Geometry check sheet. Reference: the model listing, model coordinates, mm. A direction names the side the tool comes from. Round coordinates to 2 decimals unless told otherwise and drop trailing zeros. Loops run counter-clockwise (first coordinate to the right, second up) from the corner with the lowest first, then second, coordinate; pieces in that order, holes last. Notation, with made-up numbers: (-7.75, 69) - (-3.75, 69) arc R23 cw to (-3.75, 84) - close; hole circle Ø10 at (85.5, 69.5). An arc over 180 degrees is marked (long way). Answer in a Markdown table with one row per item. Add a question column.
```python
from build123d import *

# Parameters (mm, degrees)
SKETCH1_W           = 151
SKETCH1_H           = 100
BOSS_EXTRUDE1_DEPTH = 105
SKETCH2_W           = 151
SKETCH2_H           = 100
SKETCH2_W_2         = 147
SKETCH2_H_2         = 96
CUT_EXTRUDE1_DEPTH  = 5
SKETCH3_W           = 20
SKETCH3_H           = 15
CUT_EXTRUDE2_DEPTH  = 2
SKETCH4_R           = 4
BOSS_EXTRUDE2_DEPTH = 5


with BuildPart() as part:
    # Sketch1 → Boss-Extrude1 (new body)
    with BuildSketch(Plane(origin=(0, 0, 0), x_dir=(1, 0, 0), z_dir=(0, 1, 0))):
        Rectangle(SKETCH1_W, SKETCH1_H)
    extrude(amount=BOSS_EXTRUDE1_DEPTH)

    # Sketch2 → Cut-Extrude1 (cut)
    with BuildSketch(Plane(origin=(0, 105, 0), x_dir=(1, 0, 0), z_dir=(0, 1, 0))):
        Rectangle(SKETCH2_W, SKETCH2_H)
        Rectangle(SKETCH2_W_2, SKETCH2_H_2, mode=Mode.SUBTRACT)
    extrude(amount=-CUT_EXTRUDE1_DEPTH, mode=Mode.SUBTRACT)

    # Sketch3 → Cut-Extrude2 (cut)
    with BuildSketch(Plane(origin=(0, 105, 0), x_dir=(1, 0, 0), z_dir=(0, 1, 0))):
        with Locations((63.5, 37.5)):
            Rectangle(SKETCH3_W, SKETCH3_H)
        with Locations((63.5, -37.5)):
            Rectangle(SKETCH3_W, SKETCH3_H)
    extrude(amount=-CUT_EXTRUDE2_DEPTH, mode=Mode.SUBTRACT)

    # Sketch4 → Boss-Extrude2 (add)
    with BuildSketch(Plane(origin=(0, 103, 0), x_dir=(1, 0, 0), z_dir=(0, 1, 0))):
        with Locations(Location((63.5, -37.5, 0), (0, 0, 270))):
            Circle(SKETCH4_R)
        with Locations(Location((63.5, 37.5, 0), (0, 0, 90))):
            Circle(SKETCH4_R)
    extrude(amount=BOSS_EXTRUDE2_DEPTH)


solid = part.part
```
Q1. Scan lines: line 1 (Y direction, x = 6, z = 23); line 2 (Y direction, x = 55.5, z = -32). Record each from-to range of solid material in increasing order. Write a range as from..to.
Q2. Cross-section at B-B, the plane z = -1. Enter the section's corners in (x, y).
Q3. Cross-section at A-A, the plane x = -21. Enter the section's corners in (y, z).
Q4. Depth check by flat-ended pin: P1, Ø5.5, axis at y = 103.5, z = -2, coming from the -X side; P2, Ø1.6, axis at y = 103.5, z = -41, coming from the +X side; P3, Ø0.6, axis at x = 61, y = 104, coming from the +Z side. Enter the tip coordinate at first touch or a pass-through.
Q5. Set-up check for faces 4 (the flat face through (-1, 0, -1)), 5 (the flat face through (-73.5, 103, 1)), 6 (the flat face through (61, 103, -41)), 7 (the flat face through (-1, 103, 48)), 8 (the flat face through (-1, 103, -48)): record each of +Z, -Z, +X, -X, +Y, -Y from which the full face is reachable in a straight line by a thin tool's end or side.
Q6. Cross-section at C-C, the plane x = 63.5. Enter the section's corners in (y, z).
Q7. Release check for a two-part mould opening along X. For faces 1 (the flat face through (-1, 49, -50)), 2 (the flat face through (61, 103, 34)), 3 (the flat face through (73.5, 102, 1)) record: +X half, -X half, draft (parallel to the pull), parting line (faces both ways), or undercut.
Check sheet entries:
| question | item | result |
|---|---|---|
| 1 | line 1 | 0..105 |
| 1 | line 2 | 0..103 |
| 2 | outline | (-75.5, 0) - (75.5, 0) - (75.5, 100) - (73.5, 100) - (73.5, 105) - (-73.5, 105) - (-73.5, 100) - (-75.5, 100) - close |
| 3 | outline | (0, -50) - (100, -50) - (100, -48) - (105, -48) - (105, 48) - (100, 48) - (100, 50) - (0, 50) - close |
| 4 | P1 | x = -73.5 |
| 4 | P2 | x = 73.5 |
| 4 | P3 | z = 48 |
| 5 | face 4 | +Z, -Z, +X, -X, -Y |
| 5 | face 5 | +Z, -Z, -X, +Y |
| 5 | face 6 | +Y |
| 5 | face 7 | +Z, +X, -X, +Y |
| 5 | face 8 | -Z, +X, -X, +Y |
| 6 | outline | (0, -50) - (100, -50) - (100, -48) - (105, -48) - (105, -45) - (103, -45) - (103, -41.5) - (108, -41.5) - (108, -33.5) - (103, -33.5) - (103, -30) - (105, -30) - (105, 30) - (103, 30) - (103, 33.5) - (108, 33.5) - (108, 41.5) - (103, 41.5) - (103, 45) - (105, 45) - (105, 48) - (100, 48) - (100, 50) - (0, 50) - close |
| 7 | face 1 | draft |
| 7 | face 2 | undercut |
| 7 | face 3 | +X half |
